```python
from build123d import *

# Parameters (mm, degrees)
SKETCH1_W                                            = 40
SKETCH1_H                                            = 40
BOSS_EXTRUDE1_DEPTH                                  = 10
F_6_0MM_DOWEL_HOLE1_D                                = 6
CBORE_FOR_M3_HEX_SOCKET_THIN_HEAD_CAP_SC_D           = 3.4
CBORE_FOR_M3_HEX_SOCKET_THIN_HEAD_CAP_SC_CBORE_D     = 6.5
CBORE_FOR_M3_HEX_SOCKET_THIN_HEAD_CAP_SC_CBORE_DEPTH = 2.4
TAP_DRILL_FOR_M4_TAP1_D                              = 3.3
CHAMFER1_SIZE                                        = 4
CHAMFER2_SIZE                                        = 0.6


with BuildPart() as part:
    # Sketch1 → Boss-Extrude1 (new body)
    with BuildSketch(Plane.XY):
        with Locations((20, 20)):
            Rectangle(SKETCH1_W, SKETCH1_H)
    extrude(amount=BOSS_EXTRUDE1_DEPTH)

    # Ø6.0mm Dowel Hole1 (through all)
    with Locations(Plane.XY.offset(10)):
        with Locations((20, 20)):
            Hole(F_6_0MM_DOWEL_HOLE1_D / 2)

    # CBORE for M3 Hex Socket Thin Head Cap Screw4 (through all)
    with Locations(Plane.XY.offset(10)):
        with Locations((13.504809472, 23.75), (20, 27.5), (26.495190528, 23.75), (26.495190528, 16.25), (20, 12.5), (13.504809472, 16.25)):
            CounterBoreHole(CBORE_FOR_M3_HEX_SOCKET_THIN_HEAD_CAP_SC_D / 2, CBORE_FOR_M3_HEX_SOCKET_THIN_HEAD_CAP_SC_CBORE_D / 2, CBORE_FOR_M3_HEX_SOCKET_THIN_HEAD_CAP_SC_CBORE_DEPTH)

    # Tap Drill for M4 Tap1 (through all)
    with Locations(Plane.XY.offset(10)):
        with Locations((9.393398282, 9.393398282), (9.393398282, 30.606601718), (30.606601718, 30.606601718), (30.606601718, 9.393398282)):
            Hole(TAP_DRILL_FOR_M4_TAP1_D / 2)

    # Chamfer1
    chamfer1_edges = [part.edges().sort_by_distance(p)[0] for p in [
        (0, 40, 5),
        (40, 40, 5),
        (40, 0, 5),
        (0, 0, 5),
    ]]
    chamfer(chamfer1_edges, length=CHAMFER1_SIZE)

    # Chamfer2
    chamfer2_edges = [part.edges().sort_by_distance(p)[0] for p in [
        (38, 2, 10),
        (40, 20, 10),
        (20, 0, 10),
        (0, 20, 10),
        (20, 40, 10),
        (2, 38, 10),
        (2, 2, 10),
        (38, 38, 10),
    ]]
    chamfer(chamfer2_edges, length=CHAMFER2_SIZE)


solid = part.part
```
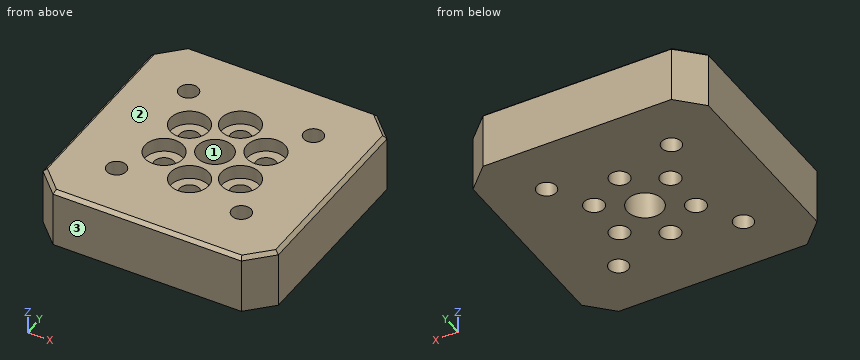
The listing builds one solid part. Answer for the finished solid, in the listing's coordinates (mm). Face numbers are marked on the shaded views. Coordinates: 2 decimals unless noted, no trailing zeros. Loops run counter-clockwise (first coordinate to the right, second up) from the corner with the lowest first, then second, coordinate; pieces in that order, holes last. Notation, with made-up numbers: (-21, -26) -> (-14, -26) arc R28 ccw to (-14, 7) -> close; hole circle Ø3 at (-35.75, -15). An arc over 180 degrees is marked (long way). Use one line per item in the form item = value. Start each with the question number.
Item 1: The part is cut by section A-A on y = 23.75. Determine the outline of the cut face in (x, z).
Item 2: The part is cut by section B-B on x = 20. Determine the outline of the cut face in (y, z), then the cut area to 3 significant figures.
Item 3: The part is cut by section D-D on z = 2.25. Count the separate pieces of the cut face and the enclosed holes in it, then the cut area to 3 significant figures.
Item 4: Consider L1, parallel to Y at x = 20, z = 8.65; L2, parallel to Y at x = 20, z = 6; L3, parallel to X at y = 9, z = 7. Determine where each line is inside the solid, lowest interval first. Write a range as [from, to].
Item 5: Flat-ended cylindrical pins translate along their axes: pin 1 Ø2.5 at (x, y) = (13.5, 16.25) entering from -Z; pin 2 Ø5 at (x, y) = (27.5, 16) entering from +Z; pin 3 Ø4 at (x, y) = (20, 12.5) entering from +Z. Find the tip coordinate at first contact, or state that the pin passes through.
Item 6: The part is cut by section C-C on y = 18.5. Determine the outline of the cut face in (x, z).
Item 7: The mould has two halves that part along Y. Classify the marked faces 1, 2 and 3: released by +Y, released by -Y, zero draft, split by the parting line, or undercut.
Answer key:
q1.outline = (0, 0) -> (11.8, 0) -> (11.8, 7.6) -> (10.25, 7.6) -> (10.25, 10) -> (0.6, 10) -> (0, 9.4) -> close; (15.2, 0) -> (24.8, 0) -> (24.8, 7.6) -> (23.25, 7.6) -> (23.25, 10) -> (16.75, 10) -> (16.75, 7.6) -> (15.2, 7.6) -> close; (28.2, 0) -> (40, 0) -> (40, 9.4) -> (39.4, 10) -> (29.75, 10) -> (29.75, 7.6) -> (28.2, 7.6) -> close
q2.outline = (0, 0) -> (10.8, 0) -> (10.8, 7.6) -> (9.25, 7.6) -> (9.25, 10) -> (0.6, 10) -> (0, 9.4) -> close; (14.2, 0) -> (17, 0) -> (17, 10) -> (15.75, 10) -> (15.75, 7.6) -> (14.2, 7.6) -> close; (23, 0) -> (25.8, 0) -> (25.8, 7.6) -> (24.25, 7.6) -> (24.25, 10) -> (23, 10) -> close; (29.2, 0) -> (40, 0) -> (40, 9.4) -> (39.4, 10) -> (30.75, 10) -> (30.75, 7.6) -> (29.2, 7.6) -> close
q2.area = 257 mm2
q3.separate_pieces = 1
q3.enclosed_holes = 11
q3.area = 1,450 mm2
q4.L1 = [0, 9.25], [15.75, 17], [23, 24.25], [30.75, 40]
q4.L2 = [0, 10.8], [14.2, 17], [23, 25.8], [29.2, 40]
q4.L3 = [0, 7.79], [11, 29], [32.21, 40]
q5.pin_1 = through
q5.pin_2 = 10
q5.pin_3 = 7.6
q6.outline = (0, 0) -> (17.4, 0) -> (17.4, 10) -> (15.85, 10) -> (15.85, 7.6) -> (11.16, 7.6) -> (11.16, 10) -> (0.6, 10) -> (0, 9.4) -> close; (22.6, 0) -> (40, 0) -> (40, 9.4) -> (39.4, 10) -> (28.84, 10) -> (28.84, 7.6) -> (24.15, 7.6) -> (24.15, 10) -> (22.6, 10) -> close
q7.face_1 = undercut
q7.face_2 = zero draft
q7.face_3 = released by -Y
